Check sheet for the modelled part. Datum: model origin and axes. Units: mm. Face numbers are marked on the shaded views. A direction names the side the tool comes from. Round coordinates to 2 decimals unless told otherwise and drop trailing zeros. Loops run counter-clockwise (first coordinate to the right, second up) from the corner with the lowest first, then second, coordinate; pieces in that order, holes last. Notation, with made-up numbers: M -8,-30.75 L -4,-30.75 A18 ccw -4,-7.75 Z; hole C 82.25,-26.75 d2. An arc over 180 degrees is marked long. One line per question, with ' | ' between items. Start each with the question number.
(1) Section check B-B (x = 12.5). Record the boundary of the cut face in (y, z).
(2) Section check C-C (z = 31). Record the boundary of the cut face in (x, y).
(3) Tool access check on the marked faces 5 and 6. Record the directions out of +Z, -Z, +X, -X, +Y, -Y that give a thin tool (end or side, any length) a straight path to the whole face; none if there is none.
(4) Section check A-A (y = -23.5). Record the boundary of the cut face in (x, z).
(5) Thickness scan on probe 1 along X at (y, z) = (-21, 9.5); probe 2 along Y at (x, z) = (16.75, -1); probe 3 along Y at (x, z) = (10.75, 15.5). Record the ranges inside material, lowest first. Write a range as [from, to].
(6) Section check D-D (x = 3.75). Record the boundary of the cut face in (y, z).
(7) Draft check along Y on the marked faces 1, 2, 3 and 4. Enter one of: +Y half, -Y half, draft (parallel to the pull), parting line (faces both ways), or undercut.
(8) Go/stop test with flat-tipped pins: P1, Ø2.5, axis at x = 13.5, y = 43.5, coming from the +Z side; P2, Ø4.5, axis at x = 12, z = 19, coming from the -Y side; P3, Ø2.5, axis at x = 12.5, z = 22.5, coming from the +Y side. Record where each tip stops, or that it passes through.
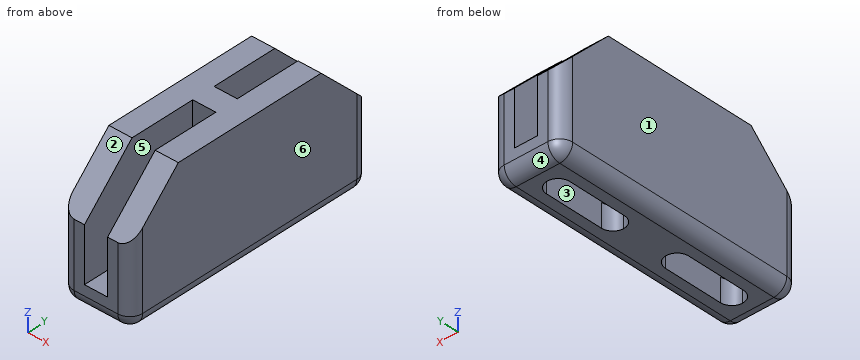
```python
from build123d import *

# Parameters (mm, degrees)
F0_W      = 41
F0_H      = 9
F1_DEPTH  = 41
F3_DEPTH  = 9
F5_DEPTH  = 9
F7_DEPTH  = 30
F9_DEPTH  = 30
F11_DEPTH = 9
F13_DEPTH = 25
F14_R     = 1
F16_W     = 18
F16_H     = 9
F17_DEPTH = 41
F19_DEPTH = 50.001
F20_R     = 5
F21_W     = 9
F21_H     = 41
F22_DEPTH = 30
F23_W     = 27
F23_H     = 9
F24_DEPTH = 41


with BuildPart() as f1:
    # F0 (on Top) → F1 (new body)
    with BuildSketch(Plane.XY):
        Polygon((0, 50), (0, 0), (27, 0), (27, 4.5), (27, 13.5), (27, 22.5), (27, 50), (18, 50), (18, 4.5), (9, 4.5), (9, 50), align=None)
        with Locations((47.5, 9)):
            Rectangle(F0_W, F0_H)
    extrude(amount=F1_DEPTH)

    # F2 (on Top) → F3 (join)
    with BuildSketch(Plane.XY):
        Polygon((0, 50), (0, 0), (68, 0), (68, 13.5), (27, 50), align=None)
    extrude(amount=-F3_DEPTH)

    # F4 (on face) → F5 (cut, through all)
    with BuildSketch(Plane.XY):
        Polygon((56.1775657399, 18), (31.5, 39.9690524269), (31.5, 18), align=None)
    extrude(amount=-F5_DEPTH, mode=Mode.SUBTRACT)

    # F6 (on face) → F7 (cut)
    with BuildSketch(Plane(origin=(0, 0, 0), x_dir=(0, -1, 0), z_dir=(-1, 0, 0))):
        Polygon((-50, 21), (-30, 41), (-50, 41), align=None)
    extrude(amount=-F7_DEPTH, mode=Mode.SUBTRACT)

    # F8 (on face) → F9 (cut)
    with BuildSketch(Plane.XZ):
        Polygon((0, 21), (0, 41), (-20, 41), align=None)
    extrude(amount=-F9_DEPTH, mode=Mode.SUBTRACT)

    # F10 (on face) → F11 (cut, through all)
    with BuildSketch(Plane.XY):
        with BuildLine():
            Line((9, 36.5), (9, 13.5))
            ThreePointArc((9, 13.5), (10.3180194847, 10.3180194847), (13.5, 9))
            ThreePointArc((13.5, 9), (16.6819805153, 10.3180194847), (18, 13.5))
            Line((18, 13.5), (18, 36.5))
            ThreePointArc((18, 36.5), (16.6819805153, 39.6819805153), (13.5, 41))
            ThreePointArc((13.5, 41), (10.3180194847, 39.6819805153), (9, 36.5))
        make_face()
        with BuildLine():
            ThreePointArc((59, 0), (57.6819805153, 3.1819805153), (54.5, 4.5))
            Line((54.5, 4.5), (40.5, 4.5))
            ThreePointArc((40.5, 4.5), (37.3180194847, 3.1819805153), (36, 0))
            Line((36, 0), (59, 0))
        make_face()
    extrude(amount=-F11_DEPTH, mode=Mode.SUBTRACT)

    # F12 (on face) → F13 (cut)
    with BuildSketch(Plane.XZ.offset(-4.5)):
        Polygon((68, 21), (68, 41), (48, 41), align=None)
        Polygon((59, 17.2720779386), (44.2720779386, 32), (36, 32), (36, 9), (59, 9), align=None)
    extrude(amount=-F13_DEPTH, mode=Mode.SUBTRACT)

    # F14
    f14_edges = [f1.edges().sort_by_distance(p)[0] for p in [
        (31.5, 18, -4.5),
        (31.5, 39.969052, -4.5),
        (56.177566, 18, -4.5),
        (36, 9, 9),
        (36, 9, 32),
        (44.272078, 9, 32),
        (59, 9, 17.272078),
        (59, 9, 9),
    ]]
    fillet(f14_edges, radius=F14_R)

    # F15: F1 across face


with BuildPart() as f1_1:
    add(f1.part)
    add(f1.part.mirror(Plane(origin=(14.5188679245, 0, 14.8396226415), x_dir=(1, 0, 0), z_dir=(0, -1, 0))))

    # F16 (on face) → F17 (cut)
    with BuildSketch(Plane.XY.offset(41)):
        with Locations((18, 0)):
            Rectangle(F16_W, F16_H)
    extrude(amount=-F17_DEPTH, mode=Mode.SUBTRACT)

    # F18 (on face) → F19 (cut, through all)
    with BuildSketch(Plane.XY.offset(41)):
        Polygon((27, 70.5021247268), (27, -13.5), (27, -65.4299333692), (95.0682684779, -18.0513188243), (92.9595008492, 35.7407592237), align=None)
    extrude(amount=-F19_DEPTH, mode=Mode.SUBTRACT)

    # F20
    f20_edges = [f1_1.edges().sort_by_distance(p)[0] for p in [
        (27, -50, 6),
        (0, -50, 6),
        (27, 50, 6),
        (0, 50, 6),
        (0, 0, -9),
        (27, 0, -9),
        (13.5, 50, -9),
        (13.5, -50, -9),
    ]]
    fillet(f20_edges, radius=F20_R)

    # F21 (on face) → F22 (cut)
    with BuildSketch(Plane.YZ.offset(27)):
        with Locations((0, 20.5)):
            Rectangle(F21_W, F21_H)
    extrude(amount=-F22_DEPTH, mode=Mode.SUBTRACT)

    # F23 (on face) → F24 (join)
    with BuildSketch(Plane.XY):
        with Locations((13.5, 0)):
            Rectangle(F23_W, F23_H)
    extrude(amount=F24_DEPTH)


solid = f1_1.part
```
The answers:
1) outline: M -50,-4 A5 ccw -45,-9 L -40.89,-9 L -40.89,0 L -50,0 Z; M -9.11,-9 L 9.11,-9 L 9.11,0 L 4.5,0 L 4.5,41 L -4.5,41 L -4.5,0 L -9.11,0 Z; M 40.89,-9 L 45,-9 A5 ccw 50,-4 L 50,0 L 40.89,0 Z
2) outline: M 0,-40 L 9,-40 L 9,-4.5 L 18,-4.5 L 18,-40 L 27,-40 L 27,40 L 18,40 L 18,4.5 L 9,4.5 L 9,40 L 0,40 Z
3) face 5: +Z | face 6: +Z, -Z, +X, +Y, -Y
4) outline: M 0,-4 A5 ccw 5,-9 L 9,-9 L 9,41 L 0,41 Z; M 18,-9 L 22,-9 A5 ccw 27,-4 L 27,41 L 18,41 Z
5) probe 1: [0, 9], [18, 27] | probe 2: [-50, -39.61], [-10.39, 10.39], [39.61, 50] | probe 3: [-4.5, 4.5]
6) outline: M -49.84,-4 A4.84 ccw -45,-8.84 L 45,-8.84 A4.84 ccw 49.84,-4 L 49.84,21.16 L 30,41 L -30,41 L -49.84,21.16 Z
7) face 1: draft | face 2: -Y half | face 3: undercut | face 4: +Y half
8) P1: z = 0 | P2: y = -4.5 | P3: y = 4.5
